Study the drawing (mm; zero at the part's minimum x, y, z) and answer. A direction names the side the tool comes from. Coordinates: 2 decimals unless noted, no trailing zeros. Order: outer loops, then holes, each group sorted by start corner. A loop starts at its lowest first (then second) coordinate and runs counter-clockwise, first axis right, second up.
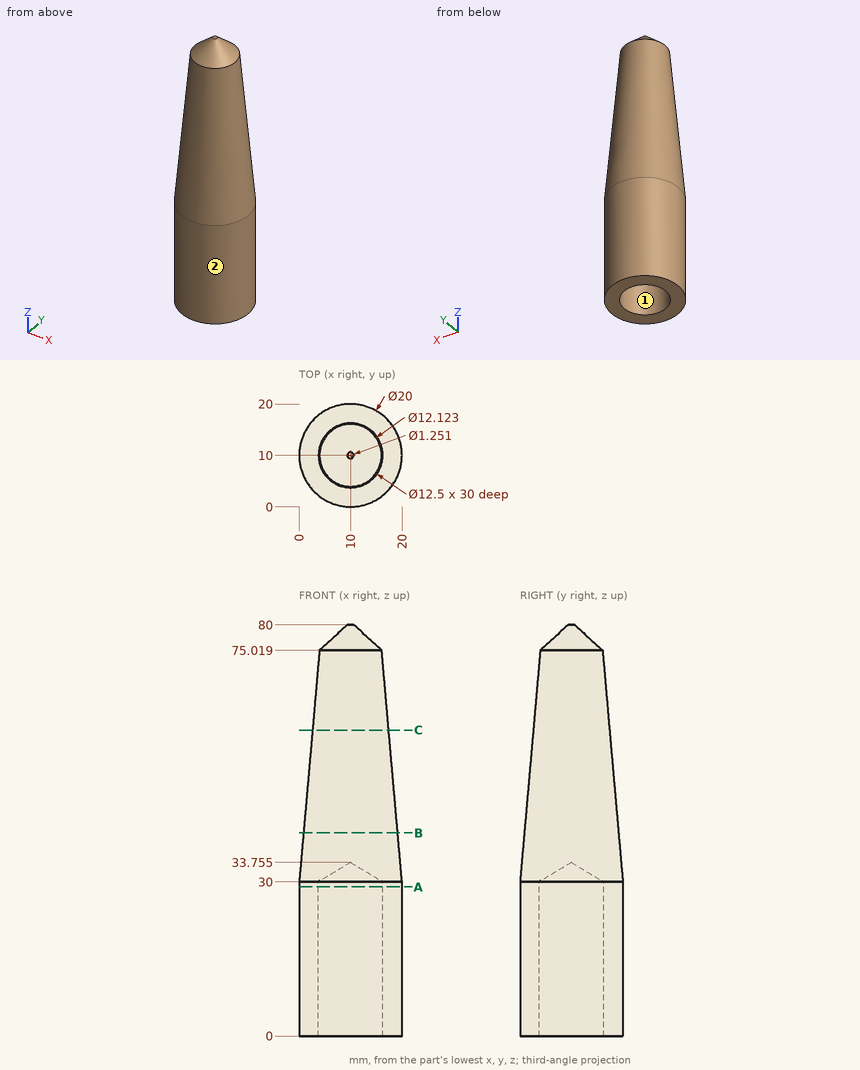
(1) Given pin 1 Ø3 at (x, y) = (9, 5.5) entering from -Z (1 decimal); pin 2 Ø1 at (y, z) = (8, 33) entering from -X; pin 3 Ø12 at (x, z) = (4.5, 40.5) entering from +Y (1 decimal), each flat-ended and moving along its own axis, determine where each tip first touches the part or whether it passes through.
(2) Find section B-B on z = 39.5. Determine the outline of the cut face in (x, y).
(3) Find section A-A on z = 29. Determine the outline of the cut face in (x, y).
(4) Find the intervals of material crossed by probe 1 along Y at (x, z) = (10, 15); probe 2 along Y at (x, z) = (6.5, 14); probe 3 along X at (y, z) = (15.75, 72.5), in increasing order.
(5) A tool of negligible diameter and unlimited length cuts with its end or side. For the marked faces 1 and 2, from which of +Z, -Z, +X, -X, +Y, -Y can it reach the whole face along a straight path? Write none if from no direction.
(6) Find section C-C on z = 59.5. Determine the outline of the cut face in (x, y), then the cut area to 3 significant figures.
Resolved:
1. pin 1: stops at z = 30.1
1. pin 2: stops at x = 0.37
1. pin 3: stops at y = 19.4
2. outline: circle Ø18.34 at (10, 10)
3. outline: circle Ø20 at (10, 10); hole circle Ø12.5 at (10, 10)
4. probe 1: y = 0 to 3.75, 16.25 to 20
4. probe 2: y = 0.63 to 4.82, 15.18 to 19.37
4. probe 3: x = 7.47 to 12.53
5. face 1: -Z
5. face 2: +Z, -Z
6. outline: circle Ø14.84 at (10, 10)
6. area: 173 mm2
